from build123d import *

# Parameters (mm, degrees)
ESBO_O1_W                = 204
ESBO_O1_H                = 120
RESSALTO_EXTRUS_O1_DEPTH = 5
ESBO_O2_W                = 5
ESBO_O2_H                = 3
ESBO_O2_W_2              = 3
ESBO_O2_H_2              = 5
RESSALTO_EXTRUS_O2_DEPTH = 5
ESBO_O3_W                = 40
ESBO_O3_H                = 20
CORTE_EXTRUS_O1_DEPTH    = 10


with BuildPart() as part:
    # Esboço1 → Ressalto-extrusão1 (new body)
    with BuildSketch(Plane.XY):
        with Locations((50.579294312, -29.131049069)):
            Rectangle(ESBO_O1_W, ESBO_O1_H)
    extrude(amount=RESSALTO_EXTRUS_O1_DEPTH)

    # Esboço2 → Ressalto-extrusão2 (add)
    with BuildSketch(Plane.XY.offset(5)):
        with Locations((50.579294312, 29.368950931)):
            Rectangle(ESBO_O2_W, ESBO_O2_H)
        with Locations((50.579294312, -87.631049069)):
            Rectangle(ESBO_O2_W, ESBO_O2_H)
        with Locations((-49.920705688, -29.131049069)):
            Rectangle(ESBO_O2_W_2, ESBO_O2_H_2)
        with Locations((151.079294312, -29.131049069)):
            Rectangle(ESBO_O2_W_2, ESBO_O2_H_2)
    extrude(amount=RESSALTO_EXTRUS_O2_DEPTH)

    # Esboço3 → Corte-extrusão1 (cut)
    with BuildSketch(Plane(origin=(0, 0, 0), x_dir=(-1, 0, 0), z_dir=(0, 0, -1))):
        with Locations((31.420705688, 20.868950931)):
            Rectangle(ESBO_O3_W, ESBO_O3_H)
    extrude(amount=-CORTE_EXTRUS_O1_DEPTH, mode=Mode.SUBTRACT)


solid = part.part
Geometry: final body of the model. Coordinates: model frame, mm. A direction names the side the tool comes from. Coordinates: 2 decimals unless noted, no trailing zeros. Order: outer loops, then holes, each group sorted by start corner. A loop starts at its lowest first (then second) coordinate and runs counter-clockwise, first axis right, second up.
(1) Section query C-C (y = -40). Return the cut outline in (x, z), plus the area to 3 significant figures.
(2) Section query B-B (x = -18). Return the cut outline in (y, z).
(3) Material intervals for probe 1 along Z at (x, y) = (14, -9); probe 2 along Y at (x, z) = (-29, 3.5), sorted ascending.
(4) Access query for faces 1 (the face through (69, 30.869, 3)), 2 (the face through (-11.421, 21, 2)), 3 (the face through (51, -86.131, 7)), 4 (the face through (149.579, -29, 7)), 5 (the face through (152.579, -30, 3)). Directions: +Z, -Z, +X, -X, +Y, -Y. A direction counts if a zero-diameter tool reaches every point of the face in a straight line with its end or side. Return the directions, or none.
(5) First-contact query: pin 1 (2 mm diameter, centred on x = 129, z = 5.5, fed in from +Y); pin 2 (1.5 mm diameter, centred on x = -49.5, z = 7.5, fed in from -Y); pin 3 (5 mm diameter, centred on x = 131.5, y = -56, fed in from +Z); pin 4 (1.5 mm diameter, centred on y = 30, z = 7, fed in from -X). Flat tips, straight axial feed; report the tip coordinate or a pass-through.
(6) Section query A-A (z = 7). Return the cut outline in (x, y).
Solution:
1. outline: (-51.42, 0) - (152.58, 0) - (152.58, 5) - (-51.42, 5) - close
1. area: 1,020 mm2
2. outline: (-89.13, 0) - (10.87, 0) - (10.87, 5) - (-89.13, 5) - close
3. probe 1: z = 0 to 5
3. probe 2: y = -89.13 to 10.87
4. face 1: +Z, -Z, +X, -X, +Y
4. face 2: +Z, -Z, -X, +Y
4. face 3: +Z, +X, -X
4. face 4: +Z, +Y, -Y
4. face 5: +Z, -Z, +X, +Y, -Y
5. pin 1: stops at y = 30.87
5. pin 2: stops at y = -31.63
5. pin 3: stops at z = 5
5. pin 4: stops at x = 48.08
6. outline: (-51.42, -31.63) - (-48.42, -31.63) - (-48.42, -26.63) - (-51.42, -26.63) - close; (48.08, -89.13) - (53.08, -89.13) - (53.08, -86.13) - (48.08, -86.13) - close; (48.08, 27.87) - (53.08, 27.87) - (53.08, 30.87) - (48.08, 30.87) - close; (149.58, -31.63) - (152.58, -31.63) - (152.58, -26.63) - (149.58, -26.63) - close
